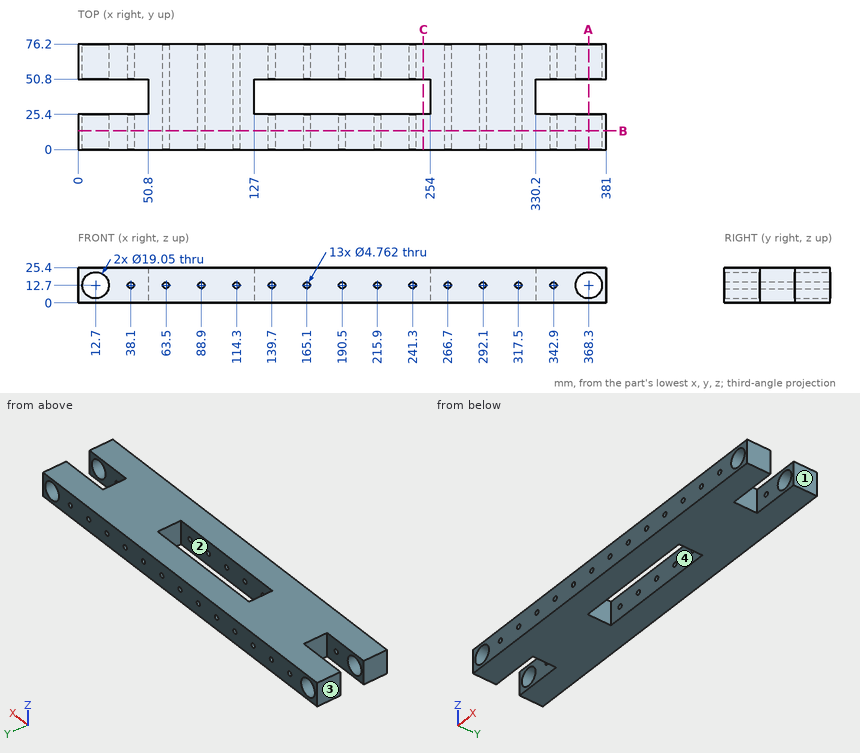
Design review of the part shown in the three views and the two pictorial views. Dimensions are in mm from the part's minimum x, y and z. Coordinates: 2 decimals unless noted, no trailing zeros. Order: outer loops, then holes, each group sorted by start corner. A loop starts at its lowest first (then second) coordinate and runs counter-clockwise, first axis right, second up.
Item 1: Take a section at B-B, the plane y = 13.5. Count the separate pieces of the cut face and the enclosed holes in it.
Item 2: The part is to be moulded in two halves that separate along X. For the marked faces 1, 2, 3 and 4, say which applies: pulls with the +X half, pulls with the -X half, needs draft (parallel to the pull), parting line crosses it, or undercut.
Item 3: Take a section at A-A, the plane x = 368.3. Write out the cut boundary in (y, z) (1 decimal).
Item 4: For pin 1 Ø4 at (x, z) = (63.5, 12.7) entering from +Y; pin 2 Ø5 at (x, z) = (301.5, 12.5) entering from -Y; pin 3 Ø8 at (y, z) = (42.5, 18) entering from -X, all flat-tipped, find the tip position at first contact; note any pin that passes through.
Item 5: Take a section at C-C, the plane x = 249. Write out the cut boundary in (y, z).
Item 6: For line 1 (Y direction, x = 44, z = 16); line 2 (X direction, y = 65, z = 5.5) (1 decimal); line 3 (X direction, y = 43, z = 19.25), list the stretches that pass through material, from the lowest coordinate up.
The answers:
1. separate pieces: 1
1. enclosed holes: 15
2. face 1: pulls with the +X half
2. face 2: undercut
2. face 3: pulls with the -X half
2. face 4: undercut
3. outline: (0, 0) - (25.4, 0) - (25.4, 3.2) - (0, 3.2) - close; (0, 22.2) - (25.4, 22.2) - (25.4, 25.4) - (0, 25.4) - close; (50.8, 0) - (76.2, 0) - (76.2, 3.2) - (50.8, 3.2) - close; (50.8, 22.2) - (76.2, 22.2) - (76.2, 25.4) - (50.8, 25.4) - close
4. pin 1: passes through
4. pin 2: stops at y = 0
4. pin 3: stops at x = 50.8
5. outline: (0, 0) - (25.4, 0) - (25.4, 25.4) - (0, 25.4) - close; (50.8, 0) - (76.2, 0) - (76.2, 25.4) - (50.8, 25.4) - close
6. line 1: y = 0 to 25.4, 50.8 to 76.2
6. line 2: x = 0 to 6.5, 18.9 to 362.1, 374.5 to 381
6. line 3: x = 50.8 to 127, 254 to 330.2
